Model file for the job. Use its own axes, mm. Round coordinates to 2 decimals unless told otherwise and drop trailing zeros. Order: outer loops, then holes, each group sorted by start corner. A loop starts at its lowest first (then second) coordinate and runs counter-clockwise, first axis right, second up. Notation, with made-up numbers: (-31, 50.25) -> (-24, 50.25) arc R31 cw to (-24, 77.25) -> close; hole circle Ø10 at (18, 58.5). An arc over 180 degrees is marked (long way). Answer as CSV lines item,"result".
Autodesk Inventor part; units mm, degrees
ref_plane "Work Plane1" through (0, 0, 0) normal (0, 0, 1) x (1, 0, 0)
ref_plane "YZ Plane" through (0, 0, 0) normal (1, 0, 0) x (0, 1, 0)
ref_plane "XZ Plane" through (0, 0, 0) normal (0, 1, 0) x (-1, 0, 0)
ref_plane "Work Plane1" through (0, 0, 0) normal (0, 0, 1) x (1, 0, 0)
sketch "Sketch1" plane through (0, 0, 0) normal (0, 0, 1) x (1, 0, 0)
  line L0 (22.8064, -35.5) -> (-89.6938, -35.5)
  line L1 (-89.6938, -35.5) -> (-89.6938, -6)
  line L2 (22.8064, -6) -> (22.8064, -35.5)
  circle A0 centre (11.5562, -18) radius 2 construction
  line L3 (-53.1938, -16) -> (-53.1938, -30) construction
  arc A1 (-56.1938, -30) -> (-53.1938, -30) centre (-54.6938, -30) ccw construction
  line L4 (-56.1938, -30) -> (-56.1938, -16) construction
  arc A2 (-53.1938, -16) -> (-56.1938, -16) centre (-54.6938, -16) ccw construction
  line L5 (7.0562, -16) -> (7.0562, -30) construction
  arc A3 (4.0562, -30) -> (7.0562, -30) centre (5.5562, -30) ccw construction
  line L6 (4.0562, -30) -> (4.0562, -16) construction
  arc A4 (7.0562, -16) -> (4.0562, -16) centre (5.5562, -16) ccw construction
  line L7 (-13.1938, -16) -> (-13.1938, -30) construction
  arc A5 (-16.1938, -30) -> (-13.1938, -30) centre (-14.6938, -30) ccw construction
  line L8 (-16.1938, -30) -> (-16.1938, -16) construction
  arc A6 (-13.1938, -16) -> (-16.1938, -16) centre (-14.6938, -16) ccw construction
  arc A7 (19.0562, -16) -> (16.0562, -16) centre (17.5562, -16) ccw construction
  line L9 (19.0562, -16) -> (19.0562, -30) construction
  arc A8 (16.0562, -30) -> (19.0562, -30) centre (17.5562, -30) ccw construction
  line L10 (16.0562, -30) -> (16.0562, -16) construction
  line L11 (22.8064, -40) -> (22.8064, 45) construction
  line L12 (22.8064, 45) -> (-120, 45) construction
  line L13 (-120, 27.5563) -> (-120, 45) construction
  line L14 (-120, 27.5563) -> (-95.2035, 27.5563) construction
  arc A9 (-85.0841, 27.5563) -> (-95.2035, 27.5563) centre (-90.1438, 25.4) ccw construction
  line L15 (-85.0841, 27.5563) -> (17.8062, 27.5563) construction
  line L16 (17.8062, 27.5563) -> (17.8062, -11) construction
  line L17 (17.8062, -11) -> (-120, -11) construction
  line L18 (-120, -40) -> (-120, -11) construction
  line L19 (22.8064, -40) -> (-120, -40) construction
  circle A10 centre (-111.1938, -18) radius 2 construction
  circle A11 centre (-98.1938, -18) radius 2 construction
  circle A12 centre (-61.1938, -18) radius 2 construction
  circle A13 centre (-48.1938, -18) radius 2 construction
  circle A14 centre (-21.1938, -18) radius 2 construction
  circle A15 centre (-8.1938, -18) radius 2 construction
  circle A16 centre (-21.1938, 33.6563) radius 2 construction
  circle A17 centre (-8.1938, 33.6563) radius 2 construction
  circle A18 centre (-61.1938, 33.6563) radius 2 construction
  circle A19 centre (-48.1938, 33.6563) radius 2 construction
  circle A20 centre (-111.1938, 33.6563) radius 2 construction
  circle A21 centre (-98.1938, 33.6563) radius 2 construction
  circle A22 centre (-90.1438, -25.4) radius 5.5 construction
  line L20 (-84.6938, 26.6563) -> (-89.6938, 26.6563) construction
  line L21 (-89.6938, 26.6563) -> (-89.6938, -11) construction
  line L22 (-84.6938, -11) -> (-89.6938, -11) construction
  line L23 (-84.6938, 26.6563) -> (-84.6938, -11) construction
  line L24 (-84.6938, 26.6563) -> (-84.6938, -11) construction
  circle A23 centre (1.3062, 0) radius 6 construction
  circle A24 centre (-68.1938, 0) radius 6 construction
  line L25 (-148.5613, 0) -> (51.3677, 0) construction
  line L26 (-89.6938, -6) -> (22.8064, -6)
  line L27 (5.3062, -57) -> (5.3062, 62) construction
  line L28 (-34.6938, -57) -> (-34.6938, 62) construction
  line L29 (-84.6938, -57) -> (-84.6938, 62) construction
  point P0 (17.5562, -31.5)
  dimension "d0" = 0
  dimension "d1" = 0
  dimension "d2" = 4
extrude "Main Body" add sketch "Sketch1" along normal blind 5
sketch "Sketch2" plane through (0, 0, 0) normal (0, 0, -1) x (-1, 0, 0)
  line L0 (56.1938, -30) -> (56.1938, -16) construction
  arc A0 (53.1938, -30) -> (56.1938, -30) centre (54.6938, -30) ccw construction
  line L1 (53.1938, -16) -> (53.1938, -30) construction
  arc A1 (56.1938, -16) -> (53.1938, -16) centre (54.6938, -16) ccw construction
  arc A2 (13.1938, -30) -> (16.1938, -30) centre (14.6938, -30) ccw construction
  line L2 (13.1938, -16) -> (13.1938, -30) construction
  arc A3 (16.1938, -16) -> (13.1938, -16) centre (14.6938, -16) ccw construction
  line L3 (16.1938, -30) -> (16.1938, -16) construction
  line L4 (14.6938, -16) -> (14.6938, -30) construction
  line L5 (54.6938, -16) -> (54.6938, -30) construction
  line L6 (14.6938, -27) -> (14.6938, -19) construction
  line L7 (13.2438, -27) -> (13.2438, -19)
  line L8 (16.1438, -19) -> (16.1438, -27)
  arc A4 (13.2438, -27) -> (16.1438, -27) centre (14.6938, -27) ccw
  arc A5 (16.1438, -19) -> (13.2438, -19) centre (14.6938, -19) ccw
  line L9 (54.6938, -27) -> (54.6938, -19) construction
  line L10 (53.2438, -27) -> (53.2438, -19)
  line L11 (56.1438, -19) -> (56.1438, -27)
  arc A6 (53.2438, -27) -> (56.1438, -27) centre (54.6938, -27) ccw
  arc A7 (56.1438, -19) -> (53.2438, -19) centre (54.6938, -19) ccw
  line L12 (14.6938, -19) -> (54.6938, -19) construction
  arc A8 (-7.0562, -30) -> (-4.0562, -30) centre (-5.5562, -30) ccw construction
  line L13 (-4.0562, -30) -> (-4.0562, -16) construction
  arc A9 (-4.0562, -16) -> (-7.0562, -16) centre (-5.5562, -16) ccw construction
  line L14 (-7.0562, -16) -> (-7.0562, -30) construction
  point P0 (0, 0)
  point P1 (14.6938, -23)
  point P2 (54.6938, -23)
  dimension "d7" = 0.05
  dimension "d8" = 0.05
  dimension "d9" = 3
extrude "Alignment Tabs" add sketch "Sketch2" along normal blind 1.8
sketch "Sketch3" plane through (0, 0, 5) normal (0, 0, -1) x (-1, 0, 0)
  circle A0 centre (61.1938, -18) radius 2 construction
  circle A1 centre (8.1938, -18) radius 2 construction
  line L0 (61.1938, -14) -> (61.1938, -22) construction
  line L1 (59.4438, -14) -> (59.4438, -22)
  line L2 (62.9438, -22) -> (62.9438, -14)
  arc A2 (62.9438, -14) -> (59.4438, -14) centre (61.1938, -14) ccw
  arc A3 (59.4438, -22) -> (62.9438, -22) centre (61.1938, -22) ccw
  line L3 (8.1938, -14) -> (8.1938, -22) construction
  line L4 (6.4438, -14) -> (6.4438, -22)
  line L5 (9.9438, -22) -> (9.9438, -14)
  arc A4 (9.9438, -14) -> (6.4438, -14) centre (8.1938, -14) ccw
  arc A5 (6.4438, -22) -> (9.9438, -22) centre (8.1938, -22) ccw
  point P0 (0, 0)
  dimension "d12" = 3.5
  dimension "d13" = 3.5
  dimension "d14" = 8
  dimension "d15" = 8
extrude "Slots for Screws M3" cut sketch "Sketch3" along normal through all
equation "\"d8\" = d7"
equation "\"d13\" = d12"
equation "\"d15\" = d14"
properties part number "Cuvette Aligner 100mm Flat Edge"
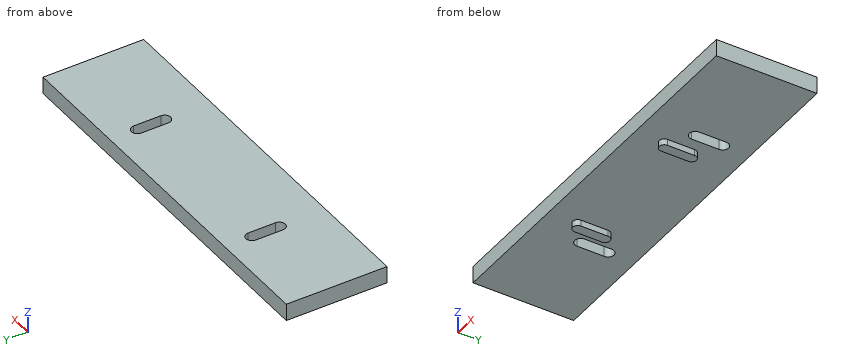
Q1. Saw through at B-B (z = 4). Write the cut outline in (x, y), plus the area to 3 significant figures.
Checks:
outline,"(-89.69, -35.5) -> (22.81, -35.5) -> (22.81, -6) -> (-89.69, -6) -> close; hole (-62.94, -22) arc R1.75 ccw to (-59.44, -22) -> (-59.44, -14) arc R1.75 ccw to (-62.94, -14) -> close; hole (-9.94, -22) arc R1.75 ccw to (-6.44, -22) -> (-6.44, -14) arc R1.75 ccw to (-9.94, -14) -> close"
area,"3,240 mm²"
Q2. Saw through at D-D (y = -10). Write the cut outline in (x, z).
Checks:
outline,"(-89.69, 0) -> (22.81, 0) -> (22.81, 5) -> (-89.69, 5) -> close"
Q3. Flat gauge pins, fed straight in: pin 1 (0.9 mm diameter, centred on y = -22, z = -1.5, fed in from -X); pin 2 (0.5 mm diameter, centred on y = -24.5, z = -0.5, fed in from +X); pin 3 (4 mm diameter, centred on x = -7.5, y = -28, fed in from -Z). Where does each tip first touch, or does it go through?
Checks:
pin 1,"x = -56.14"
pin 2,"x = -13.24"
pin 3,"z = 0"
Q4. Wall check: L1, parallel to X at y = -22.25, z = 0.5; L2, parallel to X at y = -21.5, z = 3.25; L3, parallel to Z at x = -19, y = -9.75. Give the ranges that are in metal, low to high. Write a range as [from, to].
Checks:
L1,"[-89.69, -62.93], [-59.46, -9.93], [-6.46, 22.81]"
L2,"[-89.69, -62.94], [-59.44, -9.94], [-6.44, 22.81]"
L3,"[0, 5]"
Q5. Saw through at C-C (x = 12.5). Write the cut outline in (y, z).
Checks:
outline,"(-35.5, 0) -> (-6, 0) -> (-6, 5) -> (-35.5, 5) -> close"
Q6. Saw through at A-A (y = -21). Write the cut outline in (x, z).
Checks:
outline,"(-89.69, 0) -> (-62.94, 0) -> (-62.94, 5) -> (-89.69, 5) -> close; (-59.44, 0) -> (-56.14, 0) -> (-56.14, -1.8) -> (-53.24, -1.8) -> (-53.24, 0) -> (-16.14, 0) -> (-16.14, -1.8) -> (-13.24, -1.8) -> (-13.24, 0) -> (-9.94, 0) -> (-9.94, 5) -> (-59.44, 5) -> close; (-6.44, 0) -> (22.81, 0) -> (22.81, 5) -> (-6.44, 5) -> close"
